Could you check a few things on this model? Use its own coordinates, in mm. Coordinates: 2 decimals unless noted, no trailing zeros. Loops run counter-clockwise (first coordinate to the right, second up) from the corner with the lowest first, then second, coordinate; pieces in that order, holes last. Notation, with made-up numbers: M 67.5,-6.75 L 86.5,-6.75 A27 ccw 86.5,11.25 Z; hole C 28,-36 d9. An arc over 180 degrees is marked long. Use one line per item in the form item = value. Start each with the question number.
```python
from build123d import *

# Parameters (mm, degrees)
F2_R = 5.08


with BuildPart() as f1:
    # F0 (on Front) → F1 (revolve)
    with BuildSketch(Plane.XZ):
        with BuildLine():
            Line((0, 0), (63.5, 0))
            ThreePointArc((63.5, 0), (60.2413894262, 20.0804631421), (50.8, 38.1))
            ThreePointArc((50.8, 38.1), (44.9012806053, 44.9012806053), (38.1, 50.8))
            ThreePointArc((38.1, 50.8), (20.0804631421, 60.2413894262), (0, 63.5))
            Line((0, 63.5), (0, 0))
        make_face()
        with BuildLine():
            ThreePointArc((38.1, 50.8), (44.9012806053, 44.9012806053), (50.8, 38.1))
            Line((50.8, 38.1), (76.2, 63.5))
            Line((76.2, 63.5), (76.2, 76.2))
            Line((76.2, 76.2), (63.5, 76.2))
            Line((63.5, 76.2), (38.1, 50.8))
        make_face()
    revolve(axis=Axis((0, 0, -31.75), (0, 0, -1)))

    # F2
    f2_edges = [f1.edges().sort_by_distance(p)[0] for p in [
        (-63.5, 0, 76.2),
        (-76.2, 0, 76.2),
        (-76.2, 0, 63.5),
        (-38.1, 0, 50.8),
    ]]
    fillet(f2_edges, radius=F2_R)


solid = f1.part
```
Item 1: Please list where these lines run through material, in increasing order: line 1 along Y through (x, z) = (4, 58.5) (3 decimals); line 2 along Y through (x, z) = (-18, 64.5); line 3 along Z through (x, y) = (30, -65).
Item 2: I want a section at B-B (z = 33.5). Write out the boundary of the cut face in (x, y), plus the area to 3 significant figures.
Item 3: I want a section at A-A (z = 5). Write out the boundary of the cut face in (x, y).
Item 4: I'm going to push flat-ended pins straight in: P1, Ø6, axis at y = 55, z = 25, coming from the -X side; P2, Ø5, axis at x = -8.5, z = 16, coming from the +Y side; P3, Ø1, axis at x = 12, y = -16.5, coming from the +Z side. Where does each tip first touch, or does it pass through?
Item 5: Thinking about a two-plate mould opening in X: for faces 1 (the flat face through (21, 63, 76.2)), 2 (the conical face through (49.881, -15.708, 39.596)), 3 (the conical face through (-9.13, 41.13, 54.83)), which applies, pulls with the +X half, pulls with the -X half, needs draft (parallel to the pull), parting line crosses it, or undercut?
Worked answers:
q1.line_1 = -71.088 to -45.625, -24.372 to 24.372, 45.625 to 71.088
q1.line_2 = -73.92 to -48.57, 48.57 to 73.92
q1.line_3 = 58.89 to 76.18
q2.outline = C 0,0 d107.89
q2.area = 9,140 mm²
q3.outline = C 0,0 d126.61
q4.P1 = -27.12
q4.P2 = 61.55
q4.P3 = 60.3
q5.face_1 = needs draft
q5.face_2 = parting line crosses it
q5.face_3 = undercut
